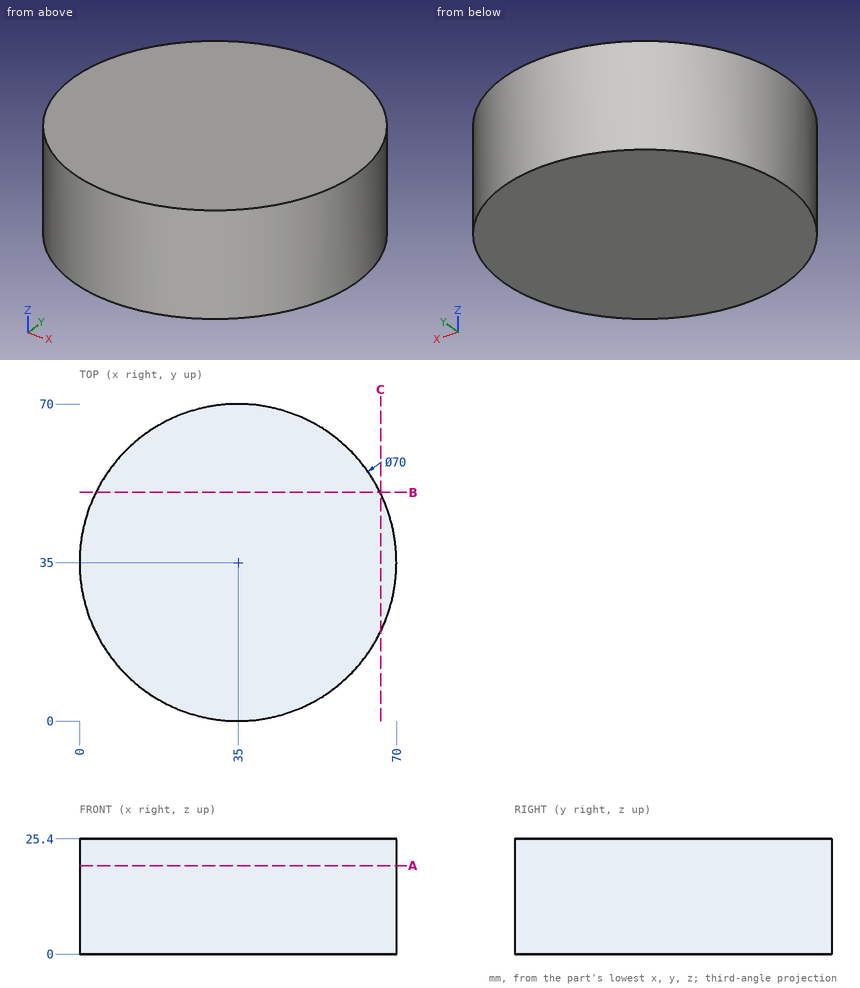
The drawing under review shows one solid part. Ordinate dimensions are in mm from its lowest x, y, z. Round coordinates to 2 decimals unless told otherwise and drop trailing zeros. Write each loop counter-clockwise with the first axis right and the second up, starting at its lowest first coordinate (ties: lowest second). Pieces come first, ordered by that corner, then holes. Notation, with made-up numbers: M 32.25,53 L 43.25,53 A12 ccw 43.25,57 Z; hole C 29,68.25 d6. An arc over 180 degrees is marked long. One line per item, written item: value. Start each with the question number.
(1) We need section C-C (x = 66.5). Give the boundary of the cut face in (y, z), and give its area (3 significant figures).
(2) Insertion check: pin 1 (12 mm diameter, centred on y = 25.5, z = 7, fed in from +X); pin 2 (10 mm diameter, centred on x = 44.5, z = 2.5, fed in from -Y); pin 3 (5 mm diameter, centred on y = 53, z = 14, fed in from -X). Each pin has a flat end and moves straight along its axis. Give the tip position at first contact, or say it passes through.
(3) We need section B-B (y = 50.5). Give the boundary of the cut face in (x, z).
(4) We need section A-A (z = 19.5). Give the boundary of the cut face in (x, y).
(5) Wall thickness on line 1 (X direction, y = 35.5, z = 11.5); line 2 (X direction, y = 19, z = 14.25); line 3 (Y direction, x = 67, z = 3.75): over which ranges is each line inside the solid? List them lowest first.
Result:
1. outline: M 19.74,0 L 50.26,0 L 50.26,25.4 L 19.74,25.4 Z
1. area: 775 mm²
2. pin 1: x = 69.82
2. pin 2: y = 0.29
2. pin 3: x = 3.62
3. outline: M 3.62,0 L 66.38,0 L 66.38,25.4 L 3.62,25.4 Z
4. outline: C 35,35 d70
5. line 1: 0 to 70
5. line 2: 3.87 to 66.13
5. line 3: 20.82 to 49.18
